Could you check a few things on this model? Use its own coordinates, in mm. A direction names the side the tool comes from. Coordinates: 2 decimals unless noted, no trailing zeros. Write each loop counter-clockwise with the first axis right and the second up, starting at its lowest first coordinate (ties: lowest second). Pieces come first, ordered by that corner, then holes. Notation, with made-up numbers: (-13, -5.5) - (-4, -5.5) arc R11 ccw to (-4, 13.5) - close; hole circle Ø8 at (-6, -18.5). An arc over 180 degrees is marked (long way). Answer as a JSON object with one key per item and string values. Group by question number.
1) If we section it at C-C (x = -27.75): Write out the boundary of the cut face in (y, z).
2) If we section it at A-A (y = 11.5): Write out the boundary of the cut face in (x, z).
3) On a 3-axis mill with a long thin cutter (end or side, diameter ignored), from which of +Z, -Z, +X, -X, +Y, -Y can I reach the whole of each face in a straight line? I mean faces 1 (the flat face through (-23.066, 7.299, 9.493)), 2 (the flat face through (-30.573, 10.2, 4.9)), 3 (the flat face through (-22.573, 4.7, 4.9)). Say none if no direction works.
4) If we section it at D-D (y = 8): Write out the boundary of the cut face in (x, z), plus the area to 3 significant figures.
5) Please list where these lines run through material, in increasing order: line 1 along X through (y, z) = (-7.15, 5); line 2 along Y through (x, z) = (-27.5, 5); line 3 along X through (y, z) = (-5.75, 3.25).
6) Will these pins go through, and if not, where does the flat tip stop? pin 1 Ø1 at (x, z) = (-32.5, 4) entering from +Y; pin 2 Ø6 at (y, z) = (7.46, 5) entering from +X; pin 3 Ø4 at (y, z) = (13, 4.5) entering from -X.
7) If we section it at B-B (z = 5): State how many separate pieces and enclosed holes the cut face has, plus the area to 3 significant figures.
8) We'd pull the mould along X, two halves only. Please class faces 4 (the cylindrical face through (-15.49, -6.28, 5.27)), 5 (the flat face through (-23.066, 7.299, 0.507)), 6 (the flat face through (-41.573, -6, 5)): released by +X, released by -X, zero draft, split by the parting line, or undercut.
```python
from build123d import *

# Parameters (mm, degrees)
EXTRUDE_1_DEPTH              = 10
CHAMFER_1_SIZE               = 2
CHAMFER_2_SIZE               = 1
CUT_EXTRUDE_2_REACH          = 21
SKETCH_3_R                   = 2.5
HOLE_WIZARD_M3_1_D           = 2.5
HOLE_WIZARD_M3_1_DEPTH       = 8
HOLE_WIZARD_M3_1_CSINK_D     = 3
HOLE_WIZARD_M3_1_CSINK_ANGLE = 90
HOLE_WIZARD_M5_1_D           = 4.2
HOLE_WIZARD_M5_1_DEPTH       = 4
HOLE_WIZARD_M5_1_CSINK_D     = 5.05
HOLE_WIZARD_M5_1_CSINK_ANGLE = 90


with BuildPart() as part:
    # 草图1 → 凸台-拉伸1 (new body)
    with BuildSketch(Plane.XY):
        Polygon((-41.573313116, -4.039574182), (-41.573313116, -8.039574182), (-11.573313116, -8.039574182), (-11.573313116, -4.039574182), (-22.573313116, -4.039574182), (-22.573313116, 18.960425818), (-30.573313116, 18.960425818), (-30.573313116, -4.039574182), align=None)
    extrude(amount=EXTRUDE_1_DEPTH)

    # 倒角1
    chamfer_1_edges = [part.edges().sort_by_distance(p)[0] for p in [
        (-11.573313116, -6.039574182, 0),
        (-41.573313116, -6.039574182, 0),
        (-11.573313116, -6.039574182, 10),
        (-41.573313116, -6.039574182, 10),
    ]]
    chamfer(chamfer_1_edges, length=CHAMFER_1_SIZE)

    # 倒角2
    chamfer_2_edges = [part.edges().sort_by_distance(p)[0] for p in [
        (-22.573313116, 7.460425818, 10),
        (-30.573313116, 7.460425818, 10),
        (-30.573313116, 7.460425818, 0),
        (-22.573313116, 7.460425818, 0),
    ]]
    chamfer(chamfer_2_edges, length=CHAMFER_2_SIZE)

    # 草图3 → 切除-拉伸2 (cut, up to next)
    with BuildSketch(Plane(origin=(-22.573313116, 0, 0), x_dir=(0, 0, -1), z_dir=(1, 0, 0)), mode=Mode.PRIVATE) as cut_extrude_2_sk1:
        with Locations((-5, 7.460425818)):
            Circle(SKETCH_3_R)
    cut_extrude_2_tool1 = extrude(cut_extrude_2_sk1.sketch, amount=-CUT_EXTRUDE_2_REACH, mode=Mode.PRIVATE) & part.part
    add(cut_extrude_2_tool1.solids().sort_by_distance((-22.573313, 7.460426, 5))[0], mode=Mode.SUBTRACT)

    # M3 螺纹孔1
    with Locations(Plane(origin=(-22.573313116, 13.960425818, 5), x_dir=(0, 0, 1), z_dir=(1, 0, 0))):
        with Locations((0, 0), (0, 13)):
            CounterSinkHole(HOLE_WIZARD_M3_1_D / 2, HOLE_WIZARD_M3_1_CSINK_D / 2, depth=HOLE_WIZARD_M3_1_DEPTH, counter_sink_angle=HOLE_WIZARD_M3_1_CSINK_ANGLE)

    # M5 螺纹孔1
    with Locations(Plane(origin=(-35.573313116, -4.039574182, 5), x_dir=(0, 0, 1), z_dir=(0, 1, 0))):
        with Locations((0, 0), (0, 18)):
            CounterSinkHole(HOLE_WIZARD_M5_1_D / 2, HOLE_WIZARD_M5_1_CSINK_D / 2, depth=HOLE_WIZARD_M5_1_DEPTH, counter_sink_angle=HOLE_WIZARD_M5_1_CSINK_ANGLE)


solid = part.part
```
Here are the results:
{
 "1": {"outline": "(-8.04, 0) - (18.96, 0) - (18.96, 10) - (-8.04, 10) - close; hole circle Ø2.5 at (0.96, 5); hole circle Ø5 at (7.46, 5); hole circle Ø2.5 at (13.96, 5)"},
 "2": {"outline": "(-30.57, 1) - (-29.57, 0) - (-23.57, 0) - (-22.57, 1) - (-22.57, 9) - (-23.57, 10) - (-29.57, 10) - (-30.57, 9) - close"},
 "3": {"face 1": "+Z, +X, +Y", "face 2": "+Z, -Z, -X, +Y", "face 3": "+Z, -Z, +X, +Y"},
 "4": {"outline": "(-30.57, 1) - (-29.57, 0) - (-23.57, 0) - (-22.57, 1) - (-22.57, 2.56) - (-30.57, 2.56) - close; (-30.57, 7.44) - (-22.57, 7.44) - (-22.57, 9) - (-23.57, 10) - (-29.57, 10) - (-30.57, 9) - close", "area": "38.9 mm²"},
 "5": {"line 1": "x = -41.57 to -37.67, -33.47 to -19.67, -15.47 to -11.57", "line 2": "y = -8.04 to -0.29, 2.21 to 4.96, 9.96 to 12.71, 15.21 to 18.96", "line 3": "x = -41.57 to -36.73, -34.41 to -18.73, -16.41 to -11.57"},
 "6": {"pin 1": "stops at y = -4.04", "pin 2": "stops at x = -22.57", "pin 3": "stops at x = -30.57"},
 "7": {"separate pieces": "6", "enclosed holes": "0", "area": "190 mm²"},
 "8": {"face 4": "undercut", "face 5": "released by +X", "face 6": "released by -X"}
}
